Drawing for the job (mm, zero at the part's lowest x, y, z). A direction names the side the tool comes from. Coordinates: 2 decimals unless noted, no trailing zeros. Write each loop counter-clockwise with the first axis right and the second up, starting at its lowest first coordinate (ties: lowest second). Pieces come first, ordered by that corner, then holes.
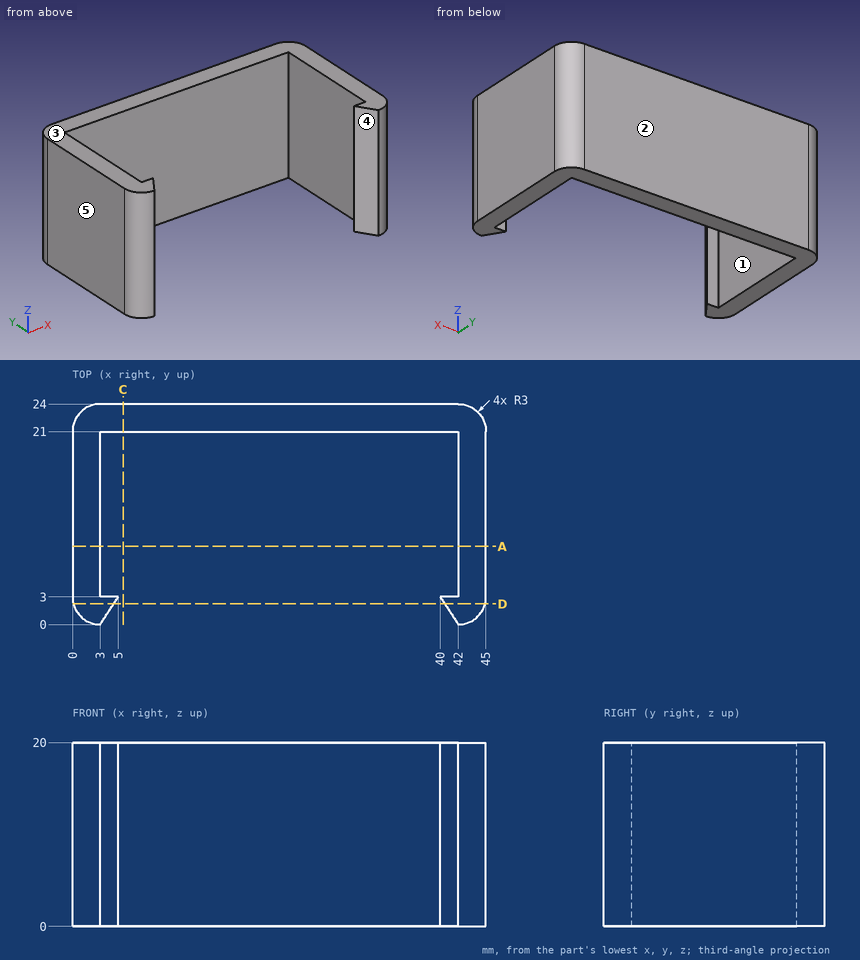
Item 1: Flat gauge pin, fed straight in: pin 1 Ø10 at (x, z) = (24.5, 8.5) entering from -Y. Where does the tip first touch, or does it go through?
Item 2: Which spindle directions (+Z, -Z, +X, -X, +Y, -Y) get a long thin tool onto all of the face, cutting with end or side? Do the marked faces 1 and 2. Say none if no direction does.
Item 3: Saw through at D-D, the plane y = 2.25. Write the cut outline in (x, z).
Item 4: Saw through at C-C, the plane x = 5.5. Write the cut outline in (y, z), and give its area (3 significant figures).
Item 5: Two-plate mould, pull along X, no slides. Class the marked faces 3, 4 and 5: +X half, -X half, draft (parallel to the pull), parting line (faces both ways), or undercut.
Item 6: Saw through at A-A, the plane y = 8.5. Write the cut outline in (x, z).
Item 7: Wall check: line 1 along X through (y, z) = (13.5, 14.25); line 2 along Y through (x, z) = (6, 13.25); line 3 along Y through (x, z) = (3.5, 3.75). Give the ranges that are in metal, low to high.
Working result:
1. pin 1: stops at y = 21
2. face 1: +Z, -Z
2. face 2: +Z, -Z, +X, -X, +Y
3. outline: (0.1, 0) - (4.5, 0) - (4.5, 20) - (0.1, 20) - close; (40.5, 0) - (44.9, 0) - (44.9, 20) - (40.5, 20) - close
4. outline: (21, 0) - (24, 0) - (24, 20) - (21, 20) - close
4. area: 60.0 mm2
5. face 3: draft
5. face 4: undercut
5. face 5: -X half
6. outline: (0, 0) - (3, 0) - (3, 20) - (0, 20) - close; (42, 0) - (45, 0) - (45, 20) - (42, 20) - close
7. line 1: x = 0 to 3, 42 to 45
7. line 2: y = 21 to 24
7. line 3: y = 0.75 to 3, 21 to 24
